from build123d import *

# Parameters (mm, degrees)
F0_R            = 2.3749
F1_DEPTH        = 6.6548
F2_R            = 4.7625
F3_DEPTH        = 5.842
F5_DEPTH        = 5.842
F5_COPIES_COUNT = 8
F7_R            = 2.921
F8_DEPTH        = 22.225


# Not quite as in the source:
# - a pattern or mirror of a feature is missing from the dataset's text; its kind, count and spacing are read off the source's solid


with BuildPart() as f1:
    # F0 (on Top) → F1 (new body)
    with BuildSketch(Plane.XY):
        with BuildLine():
            ThreePointArc((-0.1195971757, -7.2384254858), (7.0293678249, -0.1863217508), (0, 6.985))
            Line((0, 6.985), (-19.05, 6.985))
            Line((-19.05, 6.985), (-19.05, 0))
            Line((-19.05, 0), (-19.05, -7.1393631719))
            Line((-19.05, -7.1393631719), (-0.1195971757, -7.2384254858))
        make_face()
        with Locations((-0.0823807711, -0.1265228614)):
            Circle(F0_R, mode=Mode.SUBTRACT)
    extrude(amount=F1_DEPTH)

    # F2 (on Top) → F3 (join)
    with BuildSketch(Plane.XY):
        Circle(F2_R)
    extrude(amount=-F3_DEPTH)

    # F4 (on face) → F5 (cut)
    with BuildSketch(Plane(origin=(0, 0, -5.842), x_dir=(1, 0, 0), z_dir=(0, 0, -1))):
        Polygon((0, 1.3200769899), (0, 0), (0, -1.2728312286), (2.831584774, -1.2728312286), (3.7898337469, 0), (2.916136058, 1.3200769899), align=None)
    f5 = extrude(amount=-F5_DEPTH, mode=Mode.SUBTRACT)

    # F5_copies: F5 ×8 about axis
    f5_copies_axis = Axis((0, 0, 0), (0, 0, 1))
    for i in range(1, F5_COPIES_COUNT):
        add(f5.rotate(f5_copies_axis, i * 360 / F5_COPIES_COUNT), mode=Mode.SUBTRACT)

    # F7 (on offset) → F8 (cut)
    with BuildSketch(Plane.XY.offset(25.4)):
        with Locations((-0.0807045596, -0.1689054021)):
            Circle(F7_R)
    extrude(amount=-F8_DEPTH, mode=Mode.SUBTRACT)


solid = f1.part
Design review of the part built by this model. Coordinates are the model's own, in mm. A direction names the side the tool comes from. Coordinates: 2 decimals unless noted, no trailing zeros. Order: outer loops, then holes, each group sorted by start corner. A loop starts at its lowest first (then second) coordinate and runs counter-clockwise, first axis right, second up. Notation, with made-up numbers: (46, 20) -> (91, 20) arc R24 ccw to (91, 48) -> close; hole circle Ø5 at (10.25, 76). An arc over 180 degrees is marked (long way). One line per item, written item: value.
1) We need section B-B, the plane z = 5. Give the boundary of the cut face in (x, y) (3 decimals).
Output values:
outline: (-19.05, -7.139) -> (-0.12, -7.238) arc R7.112 ccw to (0, 6.985) -> (-19.05, 6.985) -> close; hole circle Ø5.842 at (-0.081, -0.169)
2) We need section C-C, the plane y = 4.5. Give the boundary of the cut face in (x, z), then the cut area to 3 significant figures.
Output values:
outline: (-19.05, 0) -> (-1.56, 0) -> (-1.56, -5.84) -> (1.56, -5.84) -> (1.56, 0) -> (5.32, 0) -> (5.32, 6.65) -> (-19.05, 6.65) -> close
area: 180 mm2
3) Clearance check with flat-ended pins moving along their axes: P1, Ø3, axis at y = -3, z = 4, coming from the +X side; P2, Ø2, axis at x = -3, z = 2.5, coming from the -Y side; P3, Ø5, axis at x = -15.5, y = 2.5, coming from the -Z side; P4, Ø3.5, axis at x = -0.08, y = -0.17, coming from the -Z side. State where each tip first meets the part, or that it passes through.
Output values:
P1: stops at x = 6.9
P2: stops at y = -7.23
P3: stops at z = 0
P4: passes through
4) We need section A-A, the plane y = -2. Give the boundary of the cut face in (x, z) (3 decimals), then the cut area to 3 significant figures.
Output values:
outline: (-19.05, 0) -> (-4.322, 0) -> (-4.322, -5.842) -> (-2.818, -5.842) -> (-2.818, 0) -> (-1.542, 0) -> (-1.542, 3.175) -> (-2.357, 3.175) -> (-2.357, 6.655) -> (-19.05, 6.655) -> close; (1.377, 0) -> (2.776, 0) -> (2.776, -5.842) -> (4.322, -5.842) -> (4.322, 0) -> (6.778, 0) -> (6.778, 6.655) -> (2.195, 6.655) -> (2.195, 3.175) -> (1.377, 3.175) -> close
area: 165 mm2
5) Machinability: for faces 4 (the face through (-9, 6.985, 3)), 5 (the face through (-0.56, 3.37, -2.96)), which of the approach directions +Z, -Z, +X, -X, +Y, -Y give a long, thin tool a straight path to every point of the face, cutting with its end or side? Answer none if there is none.
Output values:
face 4: +Z, -Z, +X, -X, +Y
face 5: -Z
6) Draft analysis for pull direction X (two halves, no side actions). For faces 1 (the face through (-19.05, 0, 3)), 2 (the face through (-3.78, -2.9, -2.88)), 3 (the face through (-2.777, 1.99, -2.962)), state which applies: +X half, -X half, draft (parallel to the pull), parting line (faces both ways), or undercut.
Output values:
face 1: -X half
face 2: parting line
face 3: undercut
7) We need section D-D, the plane y = -5.25. Give the boundary of the cut face in (x, z).
Output values:
outline: (-19.05, 0) -> (4.85, 0) -> (4.85, 6.65) -> (-19.05, 6.65) -> close
8) To check wall thickness, follow probe 1 along Z at (x, y) = (-18, 3); probe 2 along Y at (x, z) = (2.5, 3.5); probe 3 along Y at (x, z) = (-17.75, 1) (3 decimals). State the ranges of each line that lie inside material, in increasing order. Write a range as [from, to].
Output values:
probe 1: z = [0, 6.65]
probe 2: y = [-6.75, -1.54], [1.2, 6.5]
probe 3: y = [-7.146, 6.985]
